from build123d import *

# Parameters (mm, degrees)
SKETCH_1_R          = 11.05
SKETCH_1_R_2        = 2
EXTRUDE_1_DEPTH     = 36
SKETCH_3_R          = 2.5
CUT_EXTRUDE_1_DEPTH = 10


with BuildPart() as part:
    # 草图1 → 凸台-拉伸1 (new body)
    with BuildSketch(Plane.XY):
        Polygon((25, 15), (-25, 15), (-25, -8), (-13, -20), (13, -20), (25, -8), align=None)
        Circle(SKETCH_1_R, mode=Mode.SUBTRACT)
        with Locations((-16, 0)):
            Circle(SKETCH_1_R_2, mode=Mode.SUBTRACT)
        with Locations((-11.313708499, 11.313708499)):
            Circle(SKETCH_1_R_2, mode=Mode.SUBTRACT)
        with Locations((-11.313708499, -11.313708499)):
            Circle(SKETCH_1_R_2, mode=Mode.SUBTRACT)
        with Locations((11.313708499, -11.313708499)):
            Circle(SKETCH_1_R_2, mode=Mode.SUBTRACT)
        with Locations((11.313708499, 11.313708499)):
            Circle(SKETCH_1_R_2, mode=Mode.SUBTRACT)
        with Locations((16, 0)):
            Circle(SKETCH_1_R_2, mode=Mode.SUBTRACT)
    extrude(amount=EXTRUDE_1_DEPTH)

    # 草图3 → 切除-拉伸1 (cut)
    with BuildSketch(Plane(origin=(0, 15, 0), x_dir=(1, 0, 0), z_dir=(0, 1, 0))):
        with Locations((-17.5, -6)):
            Circle(SKETCH_3_R)
        with Locations((-17.5, -30)):
            Circle(SKETCH_3_R)
        with Locations((17.5, -30)):
            Circle(SKETCH_3_R)
        with Locations((17.5, -6)):
            Circle(SKETCH_3_R)
    extrude(amount=-CUT_EXTRUDE_1_DEPTH, mode=Mode.SUBTRACT)


solid = part.part
Geometry: final body of the model. Coordinates: model frame, mm. A direction names the side the tool comes from. Round coordinates to 2 decimals unless told otherwise and drop trailing zeros. Loops run counter-clockwise (first coordinate to the right, second up) from the corner with the lowest first, then second, coordinate; pieces in that order, holes last. Notation, with made-up numbers: M -3.75,-29 L 26.25,-29 A23 cw 26.25,-14 Z; hole C 34,16 d4. An arc over 180 degrees is marked long. Put each result on its own line as item: value. Start each with the question number.
(1) Material intervals for line 1 along Y through (x, z) = (0, 10); line 2 along X through (y, z) = (7.75, 6); line 3 along Y through (x, z) = (12, 19.5), sorted ascending. Write a range as [from, to].
(2) Section query B-B (y = 0). Return loops of the section in (x, z).
(3) Section query D-D (y = 4). Return loops of the section in (x, z), then the cut area to 3 significant figures.
(4) Section query A-A (x = 16). Return loops of the section in (y, z).
(5) Contact query for flat-ended pins moving along their axis: pin 1 Ø10 at (y, z) = (-12.5, 19.5) entering from +X; pin 2 Ø4 at (x, z) = (-17.5, 30) entering from +Y; pin 3 Ø8 at (x, z) = (17.5, 6) entering from -Y; pin 4 Ø5 at (x, z) = (19, 15) entering from -Y. Output: stop coordinate, or through.
(6) Draft query along X for faces 1 (the face through (-6, -10, 0)), 2 (the face through (-19, -14, 18)), 3 (the face through (16, 10, 28)). Return one class per face: +X half, -X half, draft (parallel to the pull), parting line (faces both ways), or undercut.
(7) Section query C-C (z = 30). Return loops of the section in (x, y), then the cut area to 3 significant figures.
(8) Set-up query: faces 4 (the face through (17, 5, 30)), 5 (the face through (0, 15, 18)). Return all of +Z, -Z, +X, -X, +Y, -Y with unobstructed straight access to the full face (end or side cutting, diameter ignored); none if empty.
Findings below:
1. line 1: y = [-20, -11.05], [11.05, 15]
1. line 2: x = [-25, -20], [-15, -7.88], [7.88, 15], [20, 25]
1. line 3: y = [-20, -13.19], [-9.44, 9.44], [13.19, 15]
2. outline: M -25,0 L -18,0 L -18,36 L -25,36 Z; M -14,0 L -11.05,0 L -11.05,36 L -14,36 Z; M 11.05,0 L 14,0 L 14,36 L 11.05,36 Z; M 18,0 L 25,0 L 25,36 L 18,36 Z
3. outline: M -25,0 L -10.3,0 L -10.3,36 L -25,36 Z; M 10.3,0 L 25,0 L 25,36 L 10.3,36 Z
3. area: 1,060 mm2
4. outline: M -17,0 L -2,0 L -2,36 L -17,36 Z; M 2,0 L 15,0 L 15,4 L 5,4 L 5,8 L 15,8 L 15,28 L 5,28 L 5,32 L 15,32 L 15,36 L 2,36 Z
5. pin 1: stops at x = 25
5. pin 2: stops at y = 5
5. pin 3: stops at y = -19.5
5. pin 4: stops at y = -16.5
6. face 1: draft
6. face 2: -X half
6. face 3: undercut
7. outline: M -25,-8 L -13,-20 L 13,-20 L 25,-8 L 25,15 L 20,15 L 20,5 L 15,5 L 15,15 L -15,15 L -15,5 L -20,5 L -20,15 L -25,15 Z; hole C -16,0 d4; hole C -11.31,-11.31 d4; hole C -11.31,11.31 d4; hole C 0,0 d22.1; hole C 11.31,-11.31 d4; hole C 11.31,11.31 d4; hole C 16,0 d4
7. area: 1,050 mm2
8. face 4: +Y
8. face 5: +Z, -Z, +X, -X, +Y
